The listing builds one solid part. Answer for the finished solid, in the listing's coordinates (mm). A direction names the side the tool comes from. Round coordinates to 2 decimals unless told otherwise and drop trailing zeros. Write each loop counter-clockwise with the first axis right and the second up, starting at its lowest first coordinate (ties: lowest second). Pieces come first, ordered by that corner, then holes.
Item 1: Find section B-B on y = -20.6. Give the vertices of the cut face in (x, z), then the cut area to 3 significant figures.
Item 2: Each of these flat-tipped pins is pushed along its axis until it touches: pin 1 (0.5 mm diameter, centred on x = -1.5, z = 0.5, fed in from +Y); pin 2 (1.4 mm diameter, centred on y = -9.5, z = 2.5, fed in from +X); pin 3 (0.6 mm diameter, centred on x = 0, z = 0.5, fed in from -Y); pin 4 (1.5 mm diameter, centred on x = -8, z = 6, fed in from -Y). Where does it stop, or does it pass through?
Item 3: A tool of negligible diameter and unlimited length cuts with its end or side. For faces 1 (the face through (-5.9, -9, 2)), 2 (the face through (0, -24.6, 2)), 3 (the face through (0, -16.6, 2)), 4 (the face through (-1.5, -21, 5)), from which of +Z, -Z, +X, -X, +Y, -Y can it reach the whole face along a straight path? Write none if from no direction.
Item 4: For a pull along Y with two mould halves and no side action, classify faces 5 (the face through (-1.99, -21.55, 5.87)), 6 (the face through (2.5, -21, 5)), 7 (the face through (11.85, -33.17, -0.51)) as +Y half, -Y half, draft (parallel to the pull), parting line (faces both ways), or undercut.
Item 5: Find section D-D on y = -2. Give the vertices of the cut face in (x, z).
Item 6: Find section A-A on y = -9.15. Give the vertices of the cut face in (x, z).
Item 7: Find the intervals of material crossed by probe 1 along Z at (x, y) = (-2.05, -20.6); probe 2 along Y at (x, z) = (-2, 5); probe 3 along X at (y, z) = (-9, 1.5), in increasing order.
Item 8: Find section C-C on z = 6.75. Give the vertices of the cut face in (x, y).
```python
from build123d import *

# Parameters (mm, degrees)
F0_W      = 10.85
F0_H      = 10
F0_W_2    = 2.5
F0_H_2    = 8
F0_W_3    = 7.45
F0_H_3    = 3.2
F0_H_4    = 8.5
F0_W_4    = 5.9
F1_DEPTH  = 3
F2_DEPTH  = 0.563
F3_DEPTH  = 5
F6_DEPTH  = 11.8
F7_DEPTH  = 5
F8_DEPTH  = 25
F9_R      = 2.056128731
F10_DEPTH = 1
F11_R     = 5
F12_R     = 5
F13_R     = 2
F14_DEPTH = 3


with BuildPart() as f1:
    # F0 (on Top) → F1 (new body)
    with BuildSketch(Plane.XY):
        Polygon((-5.9, -16.6), (-13.35, -16.6), (-13.35, -24.6), (-2.5, -24.6), (-2.5, -16.6), align=None)
        with Locations((-7.925, -29.6)):
            Rectangle(F0_W, F0_H)
        with Locations((1.25, -29.6)):
            Rectangle(F0_W_2, F0_H)
        with Locations((-1.25, -29.6)):
            Rectangle(F0_W_2, F0_H)
        with Locations((-1.25, -20.6)):
            Rectangle(F0_W_2, F0_H_2)
        with Locations((1.25, -20.6)):
            Rectangle(F0_W_2, F0_H_2)
        Polygon((13.35, -24.6), (13.35, -16.6), (5.9, -16.6), (2.5, -16.6), (2.5, -24.6), align=None)
        with Locations((7.925, -29.6)):
            Rectangle(F0_W, F0_H)
        Polygon((5.9, -13.4), (0, -13.4), (0, -16.6), (2.5, -16.6), (5.9, -16.6), align=None)
        with Locations((9.625, -15)):
            Rectangle(F0_W_3, F0_H_3)
        Polygon((0, -16.6), (0, -13.4), (-5.9, -13.4), (-5.9, -16.6), (-2.5, -16.6), align=None)
        with Locations((-9.625, -15)):
            Rectangle(F0_W_3, F0_H_3)
        with Locations((-9.625, -9.15)):
            Rectangle(F0_W_3, F0_H_4)
        with Locations((-2.95, -9.15)):
            Rectangle(F0_W_4, F0_H_4)
        with Locations((2.95, -9.15)):
            Rectangle(F0_W_4, F0_H_4)
        with Locations((9.625, -9.15)):
            Rectangle(F0_W_3, F0_H_4)
        with BuildLine():
            Line((13.35, -4.9), (13.35, 0))
            ThreePointArc((13.35, 0), (9.4398755288, 9.4398755288), (0, 13.35))
            Line((0, 13.35), (0, -4.9))
            Line((0, -4.9), (5.9, -4.9))
            Line((5.9, -4.9), (13.35, -4.9))
        make_face()
        with BuildLine():
            Line((0, -4.9), (0, 13.35))
            ThreePointArc((0, 13.35), (-9.4398755288, 9.4398755288), (-13.35, 0))
            Line((-13.35, 0), (-13.35, -4.9))
            Line((-13.35, -4.9), (-5.9, -4.9))
            Line((-5.9, -4.9), (0, -4.9))
        make_face()
    extrude(amount=-F1_DEPTH)

    # F0 (on Top) → F2 (join)
    with BuildSketch(Plane.XY):
        with Locations((-2.95, -9.15)):
            Rectangle(F0_W_4, F0_H_4)
        with Locations((2.95, -9.15)):
            Rectangle(F0_W_4, F0_H_4)
    extrude(amount=F2_DEPTH)

    # F0 (on Top) → F3 (join)
    with BuildSketch(Plane.XY):
        with Locations((1.25, -20.6)):
            Rectangle(F0_W_2, F0_H_2)
        with Locations((-1.25, -20.6)):
            Rectangle(F0_W_2, F0_H_2)
    extrude(amount=F3_DEPTH)

    # F5 (on face) → F6 (join)
    with BuildSketch(Plane.YZ.offset(5.9)):
        with BuildLine():
            Line((-13.4, 0.563), (-4.9, 0.563))
            ThreePointArc((-4.9, 0.563), (-9.15, 4.813), (-13.4, 0.563))
        make_face()
    extrude(amount=-F6_DEPTH)

    # F4 (on face) → F7 (join)
    with BuildSketch(Plane.YZ.offset(2.5)):
        with BuildLine():
            Line((-19.311, 5), (-16.6, 5))
            ThreePointArc((-16.6, 5), (-20.6, 9), (-24.6, 5))
            Line((-24.6, 5), (-21.889, 5))
            ThreePointArc((-21.889, 5), (-20.6, 6.289), (-19.311, 5))
        make_face()
    extrude(amount=-F7_DEPTH)

    # F4 (on face) → F8 (cut)
    with BuildSketch(Plane.YZ.offset(2.5)):
        with BuildLine():
            ThreePointArc((-21.889, 5), (-20.6, 3.711), (-19.311, 5))
            Line((-19.311, 5), (-21.889, 5))
        make_face()
        with BuildLine():
            Line((-21.889, 5), (-19.311, 5))
            ThreePointArc((-19.311, 5), (-20.6, 6.289), (-21.889, 5))
        make_face()
    extrude(amount=-F8_DEPTH, mode=Mode.SUBTRACT)

    # F9 (on face) → F10 (join)
    with BuildSketch(Plane.YZ.offset(2.5)):
        with Locations((-20.6, 5)):
            Circle(F9_R)
    extrude(amount=-F10_DEPTH)

    # F11
    f11_edges = [f1.edges().sort_by_distance(p)[0] for p in [
        (13.35, -34.6, -1.5),
    ]]
    fillet(f11_edges, radius=F11_R)

    # F12
    f12_edges = [f1.edges().sort_by_distance(p)[0] for p in [
        (-13.35, -34.6, -1.5),
    ]]
    fillet(f12_edges, radius=F12_R)

    # F13
    f13_edges = [f1.edges().sort_by_distance(p)[0] for p in [
        (0, -34.6, -3),
    ]]
    fillet(f13_edges, radius=F13_R)

    # F14 (add): a face of the model
    f14_faces = [f1.faces().sort_by_distance(p)[0] for p in [
        (1.5, -20.6, 5),
    ]]
    extrude(f14_faces, amount=F14_DEPTH)


solid = f1.part
```
Check values:
1. outline: (-13.35, -1) arc R2 ccw to (-11.35, -3) - (11.35, -3) arc R2 ccw to (13.35, -1) - (13.35, 0) - (2.5, 0) - (2.5, 9) - (-2.5, 9) - (-2.5, 6.29) - (-1.5, 6.29) - (-1.5, 3.71) - (-2.5, 3.71) - (-2.5, 0) - (-13.35, 0) - close
1. area: 121 mm2
2. pin 1: stops at y = -4.9
2. pin 2: stops at x = 5.9
2. pin 3: stops at y = -24.6
2. pin 4: passes through
3. face 1: +Z, -X, +Y, -Y
3. face 2: +Z, +X, -X, -Y
3. face 3: +Z, +X, -X
3. face 4: -X
4. face 5: undercut
4. face 6: draft
4. face 7: -Y half
5. outline: (-13.35, -1) arc R2 ccw to (-11.35, -3) - (11.35, -3) arc R2 ccw to (13.35, -1) - (13.35, 0) - (-13.35, 0) - close
6. outline: (-13.35, -1) arc R2 ccw to (-11.35, -3) - (11.35, -3) arc R2 ccw to (13.35, -1) - (13.35, 0) - (5.9, 0) - (5.9, 4.81) - (-5.9, 4.81) - (-5.9, 0) - (-13.35, 0) - close
7. probe 1: z = -3 to 3.71, 6.29 to 9
7. probe 2: y = -24.6 to -21.89, -19.31 to -16.6
7. probe 3: x = -5.9 to 5.9
8. outline: (-2.5, -24.2) - (2.5, -24.2) - (2.5, -17) - (-2.5, -17) - close
